Could you check a few things on this drawing? It's one solid part, dimensions in mm from its lowest x, y, z. Coordinates: 2 decimals unless noted, no trailing zeros. Order: outer loops, then holes, each group sorted by start corner. A loop starts at its lowest first (then second) coordinate and runs counter-clockwise, first axis right, second up. Notation, with made-up numbers: (-27, 44.25) - (28, 44.25) arc R22 ccw to (28, 81.25) - close; hole circle Ø7 at (79.5, 33). An arc over 180 degrees is marked (long way). Answer in a Markdown table with one row per item. Add a question column.
Item 1: Thinking about a two-plate mould opening in X: for the marked faces 1, 2, 3 and 4, which applies, +X half, -X half, draft (parallel to the pull), parting line (faces both ways), or undercut?
Item 2: I want a section at B-B (y = 10.75). Please give me the cut outline in (x, z).
Item 3: If I drill on line 1 along Z through (x, y) = (6, 9.5); line 2 along X through (y, z) = (8, 6); line 3 along Z through (x, y) = (5.25, 8), over which ranges is the centre line in solid material (lowest first)? Write a range as from..to.
Item 4: I want a section at A-A (x = 6). Please give me the cut outline in (y, z).
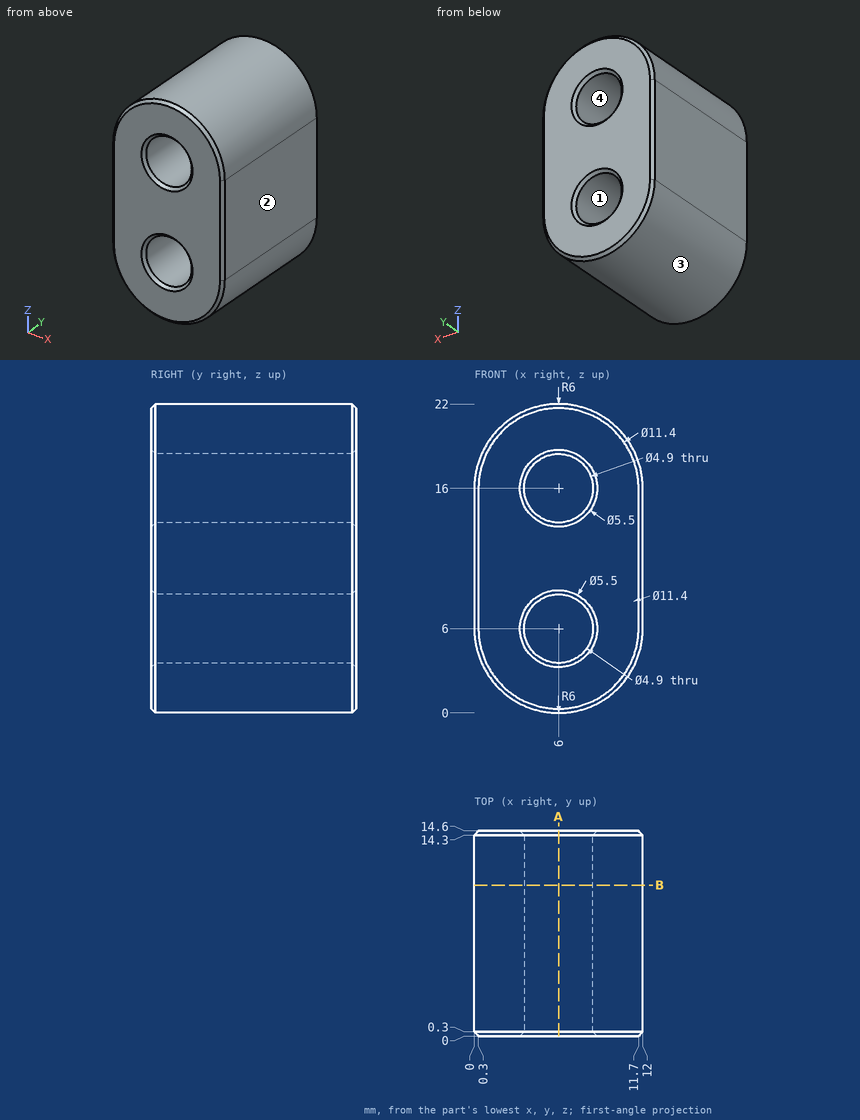
Values follow:
| question | item | result |
|---|---|---|
| 1 | face 1 | undercut |
| 1 | face 2 | +X half |
| 1 | face 3 | parting line |
| 1 | face 4 | undercut |
| 2 | outline | (0, 6) arc R6 ccw to (12, 6) - (12, 16) arc R6 ccw to (0, 16) - close; hole circle Ø4.9 at (6, 6); hole circle Ø4.9 at (6, 16) |
| 3 | line 1 | z = 0..3.55, 8.45..13.55, 18.45..22 |
| 3 | line 2 | x = 0..3.55, 8.45..12 |
| 3 | line 3 | z = 0.05..3.67, 8.33..13.67, 18.33..21.95 |
| 4 | outline | (0, 0.3) - (0.3, 0) - (14.3, 0) - (14.6, 0.3) - (14.6, 3.25) - (14.3, 3.55) - (0.3, 3.55) - (0, 3.25) - close; (0, 8.75) - (0.3, 8.45) - (14.3, 8.45) - (14.6, 8.75) - (14.6, 13.25) - (14.3, 13.55) - (0.3, 13.55) - (0, 13.25) - close; (0, 18.75) - (0.3, 18.45) - (14.3, 18.45) - (14.6, 18.75) - (14.6, 21.7) - (14.3, 22) - (0.3, 22) - (0, 21.7) - close |
